Geometry check sheet. Reference: the model listing, model coordinates, mm. Round coordinates to 2 decimals unless told otherwise and drop trailing zeros. Write each loop counter-clockwise with the first axis right and the second up, starting at its lowest first coordinate (ties: lowest second). Pieces come first, ordered by that corner, then holes. Notation, with made-up numbers: M 23,49.25 L 31,49.25 A19 cw 31,68.25 Z; hole C 8.25,7.25 d4. An arc over 180 degrees is marked long. Put each result on its own line as item: value. Start each with the question number.
(1) Section check B-B on x = 195. Record the cut outline in (y, z), then the cut area to 3 significant figures.
(2) Material ranges on probe 1 along Y at (x, z) = (49, 0.25); probe 2 along Y at (x, z) = (39.5, 2.3); probe 3 along X at (y, z) = (57.5, 0.55), recorded low to high.
(3) Section check A-A on y = 75. Record the cut outline in (x, z), then the cut area to 3 significant figures.
(4) Gauge pin test, flat ends, axial feed: pin 1 (2 mm diameter, centred on x = 211.5, z = 1, fed in from -Y); pin 2 (2 mm diameter, centred on y = 2.5, z = 2, fed in from +X); pin 3 (1.2 mm diameter, centred on y = 1.5, z = 2, fed in from +X); pin 4 (2.5 mm diameter, centred on x = 32.82, y = 96.84, fed in from +Z). Record the tip position at first contact, or that the pin passes through.
(5) Section check C-C on z = 1.25. Count the separate pieces of the cut face and the enclosed holes in it, then the cut area to 3 significant figures.
(6) Mould release check, pull along Y, two halves, no side actions. Record for faces 1 (the cylindrical face through (247.15, 146.99, 1.97)), 2 (the flat face through (123, 76, 0)), 3 (the cylindrical face through (153.54, 76.82, 2.03)): pulls with the +Y half, pulls with the -Y half, needs draft (parallel to the pull), parting line crosses it, or undercut.
from build123d import *

# Parameters (mm, degrees)
PAD001_DEPTH    = 4
SKETCH_R        = 41.5
SKETCH_R_2      = 2
SKETCH_W        = 27.573456
SKETCH_H        = 6.791874
POCKET_DEPTH    = 5
SKETCH002_W     = 20
SKETCH002_H     = 4
POCKET001_DEPTH = 5


with BuildPart() as part:
    # Sketch001 → Pad001 (new body)
    with BuildSketch(Plane.XY):
        with BuildLine():
            Line((0, 0), (240, 0))
            ThreePointArc((240, 0), (247.071068, 2.928932), (250, 10))
            Line((250, 10), (250, 140))
            ThreePointArc((250, 140), (247.071068, 147.071068), (240, 150))
            Line((240, 150), (0, 150))
            Line((0, 150), (0, 0))
        make_face()
    extrude(amount=PAD001_DEPTH)

    # Sketch (on Face8 of Pad001) → Pocket (cut)
    with BuildSketch(Plane.XY.offset(4)):
        with Locations((195, 75)):
            Circle(SKETCH_R)
        with Locations((5.433387, 53.162704)):
            Circle(SKETCH_R_2)
        with Locations((32.82399, 96.837296)):
            Circle(SKETCH_R_2)
        with Locations((32.82399, 53.162704)):
            Circle(SKETCH_R_2)
        with Locations((5.433387, 96.837296)):
            Circle(SKETCH_R_2)
        Polygon((9.23658, 112.5), (9.23658, 37.5), (29.23658, 37.5), (29.23658, 75), (29.23658, 112.5), align=None)
        with Locations((38.076655, 30.384063)):
            Rectangle(SKETCH_W, SKETCH_H)
        with Locations((38.076655, 119.615937)):
            Rectangle(SKETCH_W, SKETCH_H)
    extrude(amount=-POCKET_DEPTH, mode=Mode.SUBTRACT)

    # Sketch002 → Pocket001 (cut)
    with BuildSketch(Plane.XY):
        with Locations((10, 2)):
            Rectangle(SKETCH002_W, SKETCH002_H)
        with Locations((50, 2)):
            Rectangle(SKETCH002_W, SKETCH002_H)
        with Locations((90, 2)):
            Rectangle(SKETCH002_W, SKETCH002_H)
        with Locations((130, 2)):
            Rectangle(SKETCH002_W, SKETCH002_H)
        with Locations((170, 2)):
            Rectangle(SKETCH002_W, SKETCH002_H)
        with Locations((10, 148)):
            Rectangle(SKETCH002_W, SKETCH002_H)
        with Locations((50, 148)):
            Rectangle(SKETCH002_W, SKETCH002_H)
        with Locations((90, 148)):
            Rectangle(SKETCH002_W, SKETCH002_H)
        with Locations((130, 148)):
            Rectangle(SKETCH002_W, SKETCH002_H)
        with Locations((170, 148)):
            Rectangle(SKETCH002_W, SKETCH002_H)
        with Locations((210, 148)):
            Rectangle(SKETCH002_W, SKETCH002_H)
        with Locations((210, 2)):
            Rectangle(SKETCH002_W, SKETCH002_H)
    extrude(amount=POCKET001_DEPTH, mode=Mode.SUBTRACT)


solid = part.part
Answers follow:
1. outline: M 0,0 L 33.5,0 L 33.5,4 L 0,4 Z; M 116.5,0 L 150,0 L 150,4 L 116.5,4 Z
1. area: 268 mm^2
2. probe 1: y = 4 to 26.99, 33.78 to 116.22, 123.01 to 146
2. probe 2: y = 0 to 26.99, 33.78 to 116.22, 123.01 to 150
2. probe 3: x = 0 to 9.24, 29.24 to 157.37, 232.63 to 250
3. outline: M 0,0 L 9.24,0 L 9.24,4 L 0,4 Z; M 29.24,0 L 153.5,0 L 153.5,4 L 29.24,4 Z; M 236.5,0 L 250,0 L 250,4 L 236.5,4 Z
3. area: 588 mm^2
4. pin 1: stops at y = 4
4. pin 2: stops at x = 247.6
4. pin 3: stops at x = 246.13
4. pin 4: passes through
5. separate pieces: 1
5. enclosed holes: 8
5. area: 29,200 mm^2
6. face 1: pulls with the +Y half
6. face 2: needs draft
6. face 3: undercut
